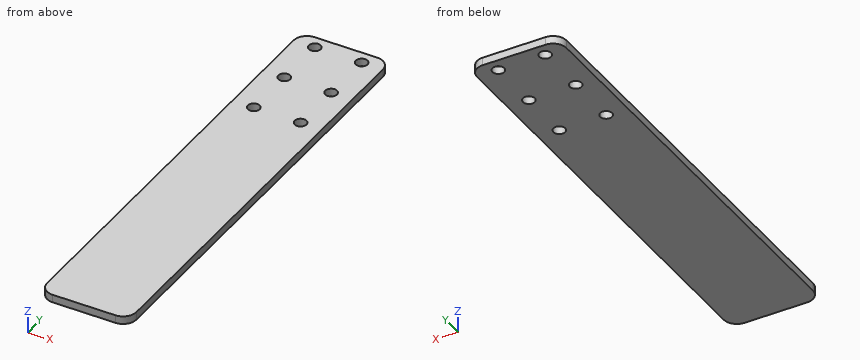
Autodesk Inventor part; units mm, degrees
ref_plane "YZ Plane" through (0, 0, 0) normal (1, 0, 0) x (0, 1, 0)
ref_plane "XZ Plane" through (0, 0, 0) normal (0, 1, 0) x (-1, 0, 0)
ref_plane "XY Plane" through (0, 0, 0) normal (0, 0, 1) x (1, 0, 0)
sketch "Block1" plane through (0, 0, 0) normal (0, 0, 1) x (1, 0, 0)
  line L0 (22.2625, 0.2735) -> (22.2625, -13.7265)
  line L1 (56.7335, -13.7265) -> (22.2625, -13.7265)
  circle A0 centre (36.0618, -8.7265) radius 2.25
  circle A1 centre (53.7335, -8.7265) radius 2.25
  line L2 (61.7335, 0.2735) -> (61.7335, -8.7265)
  arc A2 (56.7335, -13.7265) -> (61.7335, -8.7265) centre (56.7335, -8.7265) ccw
  circle A3 centre (53.7335, 11.2735) radius 2.25
  line L3 (61.7335, 20.2735) -> (61.7335, 2.2735)
  circle A4 centre (36.0618, 11.2735) radius 2.25
  line L4 (61.7335, 0.2735) -> (22.2625, 0.2735)
  line L5 (22.2625, 2.2735) -> (61.7335, 2.2735)
  line L6 (22.2625, 20.2735) -> (22.2625, 2.2735)
  line L7 (61.7335, 31.2735) -> (61.7335, 22.2735)
  line L8 (61.7335, 20.2735) -> (22.2625, 20.2735)
  line L9 (22.2625, 22.2735) -> (61.7335, 22.2735)
  circle A5 centre (36.0618, 31.2735) radius 2.25
  line L10 (56.7335, 36.2735) -> (22.2625, 36.2735)
  line L11 (22.2625, 36.2735) -> (22.2625, 22.2735)
  circle A6 centre (53.7335, 31.2735) radius 2.25
  arc A7 (61.7335, 31.2735) -> (56.7335, 36.2735) centre (56.7335, 31.2735) ccw
  point P0 (44.3211, 11.7121)
  point P1 (21.7335, 36.2735)
sketch "Sketch1" plane through (0, 0, 0) normal (0, 0, 1) x (1, 0, 0)
  line L0 (57.9999, 40.92) -> (18.5289, 40.92)
  line L1 (18.5289, 40.92) -> (18.5289, -125.6567)
  line L2 (18.5289, -125.6567) -> (57.9999, -125.6567)
  line L3 (57.9999, -125.6567) -> (57.9999, 40.92)
  line L4 (24.3282, 45.92) -> (24.3282, -125.6567)
  line L5 (18.5289, 9.92) -> (18.5289, -4.08)
  line L6 (52.9999, -4.08) -> (18.5289, -4.08)
  circle A0 centre (32.3282, 0.92) radius 2.25
  circle A1 centre (49.9999, 0.92) radius 2.25
  line L7 (57.9999, 9.92) -> (57.9999, 0.92)
  arc A2 (52.9999, -4.08) -> (57.9999, 0.92) centre (52.9999, 0.92) ccw
  circle A3 centre (49.9999, 20.92) radius 2.25
  line L8 (57.9999, 29.92) -> (57.9999, 11.92)
  circle A4 centre (32.3282, 20.92) radius 2.25
  line L9 (57.9999, 9.92) -> (18.5289, 9.92)
  line L10 (18.5289, 11.92) -> (57.9999, 11.92)
  line L11 (18.5289, 29.92) -> (18.5289, 11.92)
  line L12 (57.9999, 40.92) -> (57.9999, 31.92)
  line L13 (57.9999, 29.92) -> (18.5289, 29.92)
  line L14 (18.5289, 31.92) -> (57.9999, 31.92)
  circle A5 centre (32.3282, 40.92) radius 2.25
  line L15 (52.9999, 45.92) -> (18.5289, 45.92)
  line L16 (18.5289, 45.92) -> (18.5289, 31.92)
  circle A6 centre (49.9999, 40.92) radius 2.25
  arc A7 (57.9999, 40.92) -> (52.9999, 45.92) centre (52.9999, 40.92) ccw
  point P0 (0, 0)
  point P1 (18.5289, 40.92)
  dimension "d3" = 8
  dimension "d4" = 171.5767
extrude "Extrusion1" add sketch "Sketch1" along normal blind 3 contours L3 L14 L4 L0 A5 A6 | L0 A6 A5 L4 L15 A7 | L3 L13 L4 L14 | L3 L10 L4 L13 | L3 L9 L4 L10 | L3 A2 L6 L4 L9 | L3 L2 L4 L6 A2
fillet "Fillet1" radius 5 3 edges at (57.9999, -125.6567, 1.5) (24.3282, -125.6567, 1.5) (24.3282, 45.92, 1.5)
properties part number "Lower Leaf"
Geometry check sheet. Reference: the model listing, model coordinates, mm. Round coordinates to 2 decimals unless told otherwise and drop trailing zeros. Order: outer loops, then holes, each group sorted by start corner. A loop starts at its lowest first (then second) coordinate and runs counter-clockwise, first axis right, second up. Notation, with made-up numbers: (34, 75.25) - (55, 75.25) arc R31 cw to (55, 103.25) - close; hole circle Ø1 at (55, 57.25). An arc over 180 degrees is marked (long way). Use a Markdown table: item, result. Add a question column.
(1) Sectioned sample at B-B, the plane y = 0.92. Enter the section's corners in (x, z), and give its area (3 significant figures).
(2) Material ranges on line 1 along Y through (x, z) = (34, 0.6); line 2 along Y through (x, z) = (32, 2.45); line 3 along Y through (x, z) = (53.5, 1.65), recorded low to high. Write a range as [from, to].
(3) Depth check by flat-ended pin: pin 1 (1 mm diameter, centred on x = 45, y = -45.5, fed in from -Z); pin 2 (1.5 mm diameter, centred on x = 54, z = 1.5, fed in from -Y). Enter the tip coordinate at first touch or a pass-through.
(4) Sectioned sample at C-C, the plane z = 1.15. Enter the section's corners in (x, y), and give its area (3 significant figures).
(5) Sectioned sample at A-A, the plane x = 50.5. Enter the section's corners in (y, z).
Answers below:
| question | item | result |
|---|---|---|
| 1 | outline | (24.33, 0) - (30.08, 0) - (30.08, 3) - (24.33, 3) - close; (34.58, 0) - (47.75, 0) - (47.75, 3) - (34.58, 3) - close; (52.25, 0) - (58, 0) - (58, 3) - (52.25, 3) - close |
| 1 | area | 74.0 mm² |
| 2 | line 1 | [-125.66, -0.59], [2.43, 19.41], [22.43, 39.41], [42.43, 45.92] |
| 2 | line 2 | [-125.66, -1.31], [3.15, 18.69], [23.15, 38.69], [43.15, 45.92] |
| 2 | line 3 | [-125.63, 45.89] |
| 3 | pin 1 | z = 0 |
| 3 | pin 2 | y = -125.65 |
| 4 | outline | (24.33, -120.66) arc R5 ccw to (29.33, -125.66) - (53, -125.66) arc R5 ccw to (58, -120.66) - (58, 40.92) arc R5 ccw to (53, 45.92) - (29.33, 45.92) arc R5 ccw to (24.33, 40.92) - close; hole circle Ø4.5 at (32.33, 0.92); hole circle Ø4.5 at (32.33, 20.92); hole circle Ø4.5 at (32.33, 40.92); hole circle Ø4.5 at (50, 0.92); hole circle Ø4.5 at (50, 20.92); hole circle Ø4.5 at (50, 40.92) |
| 4 | area | 5,660 mm² |
| 5 | outline | (-125.66, 0) - (-1.27, 0) - (-1.27, 3) - (-125.66, 3) - close; (3.11, 0) - (18.73, 0) - (18.73, 3) - (3.11, 3) - close; (23.11, 0) - (38.73, 0) - (38.73, 3) - (23.11, 3) - close; (43.11, 0) - (45.92, 0) - (45.92, 3) - (43.11, 3) - close |
